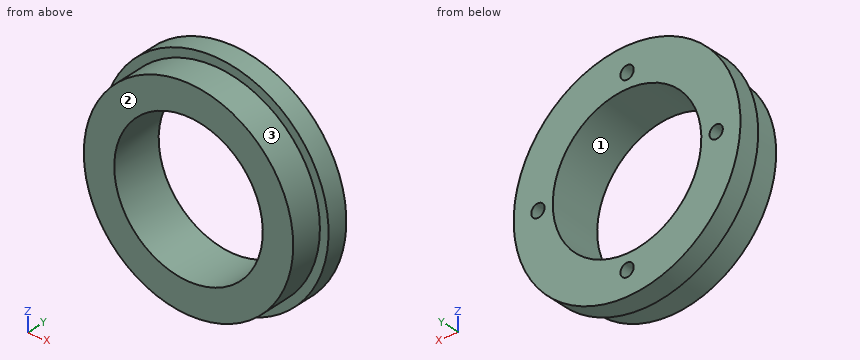
```python
from build123d import *

# Parameters (mm, degrees)
CIRPATTERN1_COUNT = 4


with BuildPart() as part:
    # Sketch1 → Revolve1 (revolve)
    with BuildSketch(Plane.XY, mode=Mode.PRIVATE) as revolve1_sk:
        Polygon((67.8561, 0), (44.45, 0), (44.45, -31.75), (62.6618, -31.75), (62.6618, -12.7), (67.8561, -12.7), align=None)
    revolve(revolve1_sk.sketch.rotate(Axis((0, -31.75, 0), (0, 1, 0)), 90), axis=Axis((0, -31.75, 0), (0, 1, 0)))

    # Sketch3 → 3/8-16 Tapped Hole1 (revolve, cut)
    with BuildSketch(Plane(origin=(0, 0, -53.34), x_dir=(0, 0, 1), z_dir=(1, 0, 0))):
        Polygon((0, 0), (0, 29.384865582), (3.96875, 27.0002), (3.96875, 0), align=None)
    f_3_8_16_tapped_hole1 = revolve(axis=Axis((0, 6.35, -53.34), (0, -1, 0)), mode=Mode.SUBTRACT)

    # CirPattern1: 3/8-16 Tapped Hole1 ×4 about axis
    cirpattern1_axis = Axis((0, 0, 0), (0, 1, 0))
    for i in range(1, CIRPATTERN1_COUNT):
        add(f_3_8_16_tapped_hole1.rotate(cirpattern1_axis, i * 360 / CIRPATTERN1_COUNT), mode=Mode.SUBTRACT)


solid = part.part
```
CAD build for the part. Positions are in the model's coordinates, mm. Face numbers are marked on the shaded views. Coordinates: 2 decimals unless noted, no trailing zeros. Write each loop counter-clockwise with the first axis right and the second up, starting at its lowest first coordinate (ties: lowest second). Pieces come first, ordered by that corner, then holes.
(1) Drill centre lines: probe 1 along X at (y, z) = (-0.5, -3); probe 2 along Z at (x, y) = (2.5, -7.5); probe 3 along X at (y, z) = (-15.5, -37). Where is each one in solid material? Low to high.
(2) Two-plate mould, pull along X, no slides. Class the marked faces 1, 2 and 3: +X half, -X half, draft (parallel to the pull), parting line (faces both ways), or undercut.
(3) Cut at B-B, the plane z = 25. List the corners of the cut face in (x, y).
(4) Cut at C-C, the plane y = -17.5. List the corners of the cut face in (x, z).
(5) Cut at A-A, the plane x = -38.5. List the corners of the cut face in (y, z).
(6) Flat gauge pins, fed straight in: pin 1 (10 mm diameter, centred on x = -42, y = -25.5, fed in from +Z); pin 2 (10 mm diameter, centred on x = -23, z = -27, fed in from -Y); pin 3 (4 mm diameter, centred on y = -11.5, z = -19.5, fed in from +X); pin 4 (4 mm diameter, centred on y = -24.5, z = 10.5, fed in from -X). Where does each tip first touch, or does it go through?
Geometry says:
1. probe 1: x = -67.79 to -55.94, -50.74 to -44.35, 44.35 to 50.74, 55.94 to 67.79
1. probe 2: z = -67.81 to -56.42, -50.26 to -44.38, 44.38 to 50.26, 56.42 to 67.81
1. probe 3: x = -50.57 to -24.63, 24.63 to 50.57
2. face 1: undercut
2. face 2: draft
2. face 3: parting line
3. outline: (-63.08, -12.7) - (-57.46, -12.7) - (-57.46, -31.75) - (-36.75, -31.75) - (-36.75, 0) - (-63.08, 0) - close; (36.75, -31.75) - (57.46, -31.75) - (57.46, -12.7) - (63.08, -12.7) - (63.08, 0) - (36.75, 0) - close
4. outline: circle Ø125.32 at (0, 0); hole circle Ø7.94 at (-53.34, 0); hole circle Ø88.9 at (0, 0); hole circle Ø7.94 at (0, -53.34); hole circle Ø7.94 at (0, 53.34); hole circle Ø7.94 at (53.34, 0)
5. outline: (-31.75, -49.44) - (-12.7, -49.44) - (-12.7, -55.88) - (0, -55.88) - (0, -22.22) - (-31.75, -22.22) - close; (-31.75, 22.22) - (0, 22.22) - (0, 55.88) - (-12.7, 55.88) - (-12.7, 49.44) - (-31.75, 49.44) - close
6. pin 1: stops at z = 50.57
6. pin 2: passes through
6. pin 3: stops at x = 65.56
6. pin 4: stops at x = -62.08
